Here's how the part is built. I have some questions about the finished solid (model axes, mm). A direction names the side the tool comes from. Coordinates: 2 decimals unless noted, no trailing zeros. Write each loop counter-clockwise with the first axis right and the second up, starting at its lowest first coordinate (ties: lowest second). Pieces come first, ordered by that corner, then holes.
```python
from build123d import *

# Parameters (mm, degrees)
SKETCH2_R          = 3
SKETCH2_R_2        = 1.5
CUT_EXTRUDE1_DEPTH = 11.31875


with BuildPart() as part:
    # Sketch1 → Revolve1 (revolve)
    with BuildSketch(Plane.XY):
        Polygon((-2.5, 20), (-10.31875, 20), (-10.31875, 0), (-5, 0), (-5, 10), (-2.5, 10), align=None)
    revolve(axis=Axis((0, 0, 0), (0, 1, 0)))

    # Sketch2 → Cut-Extrude1 (cut, through all)
    with BuildSketch(Plane.XY):
        with Locations((0, 5)):
            Circle(SKETCH2_R)
        with Locations((0, 15)):
            Circle(SKETCH2_R_2)
    extrude(amount=CUT_EXTRUDE1_DEPTH, mode=Mode.SUBTRACT)


solid = part.part
```
1) Imagine slicing it at B-B on x = 0. Please give me the cut outline in (y, z), then the cut area to 3 significant figures.
Values follow:
outline: (0, -10.32) - (20, -10.32) - (20, -2.5) - (10, -2.5) - (10, -5) - (0, -5) - close; (0, 5) - (2, 5) - (2, 10.32) - (0, 10.32) - close; (8, 5) - (10, 5) - (10, 2.5) - (13.5, 2.5) - (13.5, 10.32) - (8, 10.32) - close; (16.5, 2.5) - (20, 2.5) - (20, 10.32) - (16.5, 10.32) - close
area: 207 mm2
2) Will these pins go through, and if not, where does the flat tip stop? pin 1 (2 mm diameter, centred on y = 5.5, z = -7.5, fed in from -X); pin 2 (3 mm diameter, centred on x = 2.5, y = 11, fed in from +Z); pin 3 (1.8 mm diameter, centred on x = 0, y = 15, fed in from +Z); pin 4 (4 mm diameter, centred on x = 0, z = 0, fed in from +Y).
Values follow:
pin 1: stops at x = -8.01
pin 2: stops at z = 10.27
pin 3: stops at z = -2.33
pin 4: passes through
3) Imagine slicing it at D-D on x = -4. Please give me the cut outline in (y, z), then the cut area to 3 significant figures.
Values follow:
outline: (0, -9.51) - (20, -9.51) - (20, 9.51) - (0, 9.51) - (0, 3) - (10, 3) - (10, -3) - (0, -3) - close
area: 320 mm2
4) Imagine slicing it at C-C on y = 8.5. Please give me the cut outline in (x, z).
Values follow:
outline: circle Ø20.64 at (0, 0); hole circle Ø10 at (0, 0)
5) We'd pull the mould along X, two halves only. Please class faces 4 (the face through (1.386, 14.425, 6.103)), 5 (the face through (2.237, 9.86, -10.073)), 6 (the face through (5, 0, -2)): pulls with the +X half, pulls with the -X half, needs draft (parallel to the pull), parting line crosses it, or undercut.
Values follow:
face 4: undercut
face 5: parting line crosses it
face 6: needs draft
6) Imagine slicing it at A-A on z = 0. Please give me the cut outline in (x, y).
Values follow:
outline: (-10.32, 0) - (-5, 0) - (-5, 10) - (-2.5, 10) - (-2.5, 20) - (-10.32, 20) - close; (2.5, 10) - (5, 10) - (5, 0) - (10.32, 0) - (10.32, 20) - (2.5, 20) - close
7) I need wall thicknesses on probe 1 along Y at (x, z) = (0, 8.25); probe 2 along Z at (x, y) = (-0.25, 9.5); probe 3 along Y at (x, z) = (-1.5, -2.25). Which ranges of each line are inside material? Lowest first, please.
Values follow:
probe 1: y = 0 to 2, 8 to 13.5, 16.5 to 20
probe 2: z = -10.32 to -4.99, 4.99 to 10.32
probe 3: y = 10 to 20
8) On a 3-axis mill with a long thin cutter (end or side, diameter ignored), from which of +Z, -Z, +X, -X, +Y, -Y can I reach the whole of each face in a straight line? I mean faces 1 (the face through (-0.65, 2.07, 7.13)), 2 (the face through (1.08, 5.07, -4.88)), 3 (the face through (0.54, 15.07, -2.44)). Say none if no direction works.
Values follow:
face 1: +Z
face 2: -Y
face 3: +Y, -Y
